The model under review builds one solid part; all positions refer to its coordinate system, in mm. A direction names the side the tool comes from. Coordinates: 2 decimals unless noted, no trailing zeros. Write each loop counter-clockwise with the first axis right and the second up, starting at its lowest first coordinate (ties: lowest second). Pieces come first, ordered by that corner, then holes.
```python
from build123d import *

# Parameters (mm, degrees)
SKETCH3_W                      = 96
SKETCH3_H                      = 64
BOSS_EXTRUDE1_DEPTH            = 10
CUT_EXTRUDE1_DEPTH             = 10
SKETCH5_W                      = 16
SKETCH5_H                      = 48
BOSS_EXTRUDE2_DEPTH            = 64
CUT_EXTRUDE5_REACH             = 131.136
CUT_EXTRUDE5_DIRECTION_2_DEPTH = 130.135587659
BOSS_EXTRUDE3_START            = -64
BOSS_EXTRUDE3_DEPTH            = 42
BOSS_EXTRUDE4_DEPTH            = 12


with BuildPart() as part:
    # Sketch3 → Boss-Extrude1 (new body)
    with BuildSketch(Plane(origin=(0, 0, 0), x_dir=(1, 0, 0), z_dir=(0, 1, 0))):
        with Locations((48, 32)):
            Rectangle(SKETCH3_W, SKETCH3_H)
    extrude(amount=BOSS_EXTRUDE1_DEPTH)

    # Sketch4 → Cut-Extrude1 (cut)
    with BuildSketch(Plane(origin=(0, 10, 0), x_dir=(1, 0, 0), z_dir=(0, 1, 0))):
        with BuildLine():
            Line((96, 15.550922522), (96, 31.550922522))
            Line((96, 31.550922522), (75.043299742, 31.550922522))
            ThreePointArc((75.043299742, 31.550922522), (67.043299742, 23.550922522), (75.043299742, 15.550922522))
            Line((75.043299742, 15.550922522), (96, 15.550922522))
        make_face()
    extrude(amount=-CUT_EXTRUDE1_DEPTH, mode=Mode.SUBTRACT)

    # Sketch5 → Boss-Extrude2 (add, through all)
    with BuildSketch(Plane.XY):
        with Locations((8, 34)):
            Rectangle(SKETCH5_W, SKETCH5_H)
    extrude(amount=-BOSS_EXTRUDE2_DEPTH)

    # Sketch6 → Cut-Extrude5 (cut, up to next)
    with BuildSketch(Plane(origin=(0, 0, 0), x_dir=(0, 0, -1), z_dir=(1, 0, 0)), mode=Mode.PRIVATE) as cut_extrude5_sk1:
        with BuildLine():
            Line((0, 58), (0, 10))
            ThreePointArc((0, 10), (14.058874503, 43.941125497), (48, 58))
            Line((48, 58), (0, 58))
        make_face()
    cut_extrude5_tool1 = extrude(cut_extrude5_sk1.sketch, amount=CUT_EXTRUDE5_REACH, mode=Mode.PRIVATE) & part.part
    add(cut_extrude5_tool1.solids().sort_by_distance((0, 47.278339, -10.721661))[0], mode=Mode.SUBTRACT)

    # Sketch6 → Cut-Extrude5 direction 2 (cut)
    with BuildSketch(Plane(origin=(0, 0, 0), x_dir=(0, 0, -1), z_dir=(1, 0, 0))):
        with BuildLine():
            Line((0, 58), (0, 10))
            ThreePointArc((0, 10), (14.058874503, 43.941125497), (48, 58))
            Line((48, 58), (0, 58))
        make_face()
    extrude(amount=-CUT_EXTRUDE5_DIRECTION_2_DEPTH, mode=Mode.SUBTRACT)

    # Sketch8 → Boss-Extrude3 (add)
    with BuildSketch(Plane.XY.offset(BOSS_EXTRUDE3_START)):
        with BuildLine():
            Line((16, 10), (16, 38))
            Line((16, 38), (24, 38))
            ThreePointArc((24, 38), (36, 26), (48, 38))
            Line((48, 38), (56, 38))
            Line((56, 38), (56, 10))
            Line((56, 10), (16, 10))
        make_face()
    extrude(amount=BOSS_EXTRUDE3_DEPTH)

    # Sketch10 → Boss-Extrude4 (add)
    with BuildSketch(Plane(origin=(0, 0, -64), x_dir=(-1, 0, 0), z_dir=(0, 0, -1))):
        Polygon((-56, 38), (-96, 10), (-56, 10), align=None)
    extrude(amount=-BOSS_EXTRUDE4_DEPTH)


solid = part.part
```
Item 1: Machinability: for faces 1 (the face through (8, 58, -56)), 2 (the face through (67, 18, -52)), 3 (the face through (52, 38, -43)), 4 (the face through (86, 5, -31.551)), which of the approach directions +Z, -Z, +X, -X, +Y, -Y give a long, thin tool a straight path to every point of the face, cutting with its end or side? Answer none if there is none.
Solved:
face 1: +Z, -Z, +X, -X, +Y
face 2: +Z, +X, +Y
face 3: +Z, -Z, +X, +Y
face 4: +X, +Y, -Y
Item 2: Mouldability with a two-part tool opening along Z and no side actions: class faces 5 (the face through (67.045, 5.07, -23.727)), 6 (the face through (47, 5, 0)), 7 (the face through (0, 29, -32)) as pulls with the +Z half, pulls with the -Z half, needs draft (parallel to the pull), parting line crosses it, or undercut.
Solved:
face 5: undercut
face 6: pulls with the +Z half
face 7: needs draft
Item 3: Take a section at D-D, the plane x = 65. Write out the cut boundary in (y, z).
Solved:
outline: (0, -64) - (31.7, -64) - (31.7, -52) - (10, -52) - (10, 0) - (0, 0) - close
Item 4: Take a section at A-A, the plane z = -56.5. Write out the cut boundary in (x, y), plus the area to 3 significant figures.
Solved:
outline: (0, 0) - (96, 0) - (96, 10) - (56, 38) - (48, 38) arc R12 cw to (24, 38) - (16, 38) - (16, 58) - (0, 58) - close
area: 3,180 mm2
Item 5: To check wall thickness, follow line 1 along Y through (x, z) = (30.5, -20); line 2 along Z through (x, y) = (61, 25.5); line 3 along X through (y, z) = (32, -6). State the ranges of each line that lie inside material, in increasing order.
Solved:
line 1: y = 0 to 10
line 2: z = -64 to -52
line 3: x = 0 to 16
Item 6: Take a section at C-C, the plane y = 22.5. Write out the cut boundary in (x, z), plus the area to 3 significant figures.
Solved:
outline: (0, -64) - (78.14, -64) - (78.14, -52) - (56, -52) - (56, -22) - (16, -22) - (16, -1.66) - (0, -1.66) - close
area: 2,940 mm2
Item 7: For pin 1 (6.5 mm diameter, centred on x = 54, z = -49, fed in from +Y); pin 2 (3 mm diameter, centred on x = 18.5, y = 52, fed in from -Z); pin 3 (24 mm diameter, centred on y = 30.5, z = -18.5, fed in from +X); pin 4 (1.5 mm diameter, centred on x = 61.5, z = -49, fed in from +Y), all flat-tipped, find the tip position at first contact; note any pin that passes through.
Solved:
pin 1: stops at y = 38
pin 2: passes through
pin 3: stops at x = 56
pin 4: stops at y = 10
Item 8: Take a section at B-B, the plane x = 49.5. Write out the cut boundary in (y, z), plus the area to 3 significant figures.
Solved:
outline: (0, -64) - (38, -64) - (38, -22) - (10, -22) - (10, 0) - (0, 0) - close
area: 1,820 mm2
